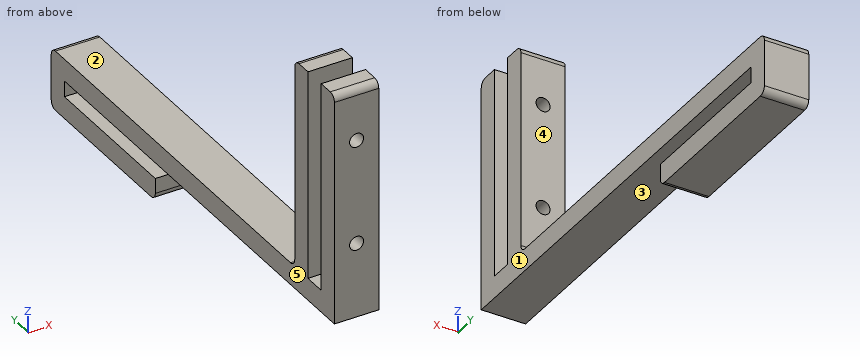
from build123d import *

# Parameters (mm, degrees)
SKETCH1_W           = 12.7
SKETCH1_H           = 66.548
BOSS_EXTRUDE1_DEPTH = 6.35
SKETCH2_W           = 12.7
SKETCH2_H           = 6.35
BOSS_EXTRUDE2_DEPTH = 6.35
SKETCH3_W           = 12.7
SKETCH3_H           = 66.548
BOSS_EXTRUDE3_DEPTH = 6.35
SKETCH4_W           = 12.7
SKETCH4_H           = 6.35
BOSS_EXTRUDE4_DEPTH = 117
SKETCH5_W           = 12.7
SKETCH5_H           = 6.35
BOSS_EXTRUDE5_DEPTH = 4.572
SKETCH6_W           = 12.7
SKETCH6_H           = 50
BOSS_EXTRUDE6_DEPTH = 6.35
BOSS_EXTRUDE7_DEPTH = 6.35
SKETCH9_R           = 2
CUT_EXTRUDE1_DEPTH  = 141.896738429
FILLET1_R           = 2
FILLET2_R           = 2


with BuildPart() as part:
    # Sketch1 → Boss-Extrude1 (new body)
    with BuildSketch(Plane(origin=(0, 0, 0), x_dir=(1, 0, 0), z_dir=(0, 1, 0))):
        with Locations((6.35, 33.274)):
            Rectangle(SKETCH1_W, SKETCH1_H)
    extrude(amount=BOSS_EXTRUDE1_DEPTH)

    # Sketch2 → Boss-Extrude2 (add)
    with BuildSketch(Plane(origin=(0, 6.35, 0), x_dir=(1, 0, 0), z_dir=(0, 1, 0))):
        with Locations((6.35, 63.373)):
            Rectangle(SKETCH2_W, SKETCH2_H)
    extrude(amount=BOSS_EXTRUDE2_DEPTH)

    # Sketch3 → Boss-Extrude3 (add)
    with BuildSketch(Plane(origin=(0, 12.7, 0), x_dir=(1, 0, 0), z_dir=(0, 1, 0))):
        with Locations((6.35, 33.274)):
            Rectangle(SKETCH3_W, SKETCH3_H)
    extrude(amount=BOSS_EXTRUDE3_DEPTH)

    # Sketch4 → Boss-Extrude4 (add)
    with BuildSketch(Plane(origin=(0, 19.05, 0), x_dir=(1, 0, 0), z_dir=(0, 1, 0))):
        with Locations((6.35, 63.373)):
            Rectangle(SKETCH4_W, SKETCH4_H)
    extrude(amount=BOSS_EXTRUDE4_DEPTH)

    # Sketch5 → Boss-Extrude5 (add)
    with BuildSketch(Plane(origin=(0, 0, -66.548), x_dir=(-1, 0, 0), z_dir=(0, 0, -1))):
        with Locations((-6.35, 132.875)):
            Rectangle(SKETCH5_W, SKETCH5_H)
    extrude(amount=BOSS_EXTRUDE5_DEPTH)

    # Sketch6 → Boss-Extrude6 (add)
    with BuildSketch(Plane(origin=(0, 0, -71.12), x_dir=(-1, 0, 0), z_dir=(0, 0, -1))):
        with Locations((-6.35, 111.05)):
            Rectangle(SKETCH6_W, SKETCH6_H)
    extrude(amount=BOSS_EXTRUDE6_DEPTH)

    # Sketch7 → Boss-Extrude7 (add)
    with BuildSketch(Plane(origin=(0, 6.35, 0), x_dir=(1, 0, 0), z_dir=(0, 1, 0))):
        with BuildLine():
            Line((12.7, 60.198), (0, 60.198))
            ThreePointArc((0, 60.198), (6.35, 60.107267194), (12.7, 60.198))
        make_face()
    extrude(amount=BOSS_EXTRUDE7_DEPTH)

    # Sketch9 → Cut-Extrude1 (cut, through all)
    with BuildSketch(Plane(origin=(0, 19.05, 0), x_dir=(1, 0, 0), z_dir=(0, 1, 0))):
        with Locations(Location((6.35, 45.099, 0), (0, 0, 270))):
            Circle(SKETCH9_R)
        with Locations(Location((6.35, 15.099, 0), (0, 0, 270))):
            Circle(SKETCH9_R)
    extrude(amount=-CUT_EXTRUDE1_DEPTH, mode=Mode.SUBTRACT)

    # Fillet1
    fillet1_edges = [part.edges().sort_by_distance(p)[0] for p in [
        (6.35, 19.05, 0),
        (6.35, 136.05, -60.198),
        (6.35, 0, 0),
        (6.35, 86.05, -77.47),
        (6.35, 136.05, -77.47),
    ]]
    fillet(fillet1_edges, radius=FILLET1_R)

    # Fillet2
    fillet2_edges = [part.edges().sort_by_distance(p)[0] for p in [
        (6.35, 19.05, -60.198),
    ]]
    fillet(fillet2_edges, radius=FILLET2_R)


solid = part.part
For this review, take the finished solid that the model builds, in its own axes (mm). Face numbers are marked on the shaded views. A direction names the side the tool comes from. Give positions to 0.01 mm unless a question says otherwise; leave off trailing zeros. Order: outer loops, then holes, each group sorted by start corner. A loop starts at its lowest first (then second) coordinate and runs counter-clockwise, first axis right, second up. Notation, with made-up numbers: (65, 0) -> (88, 0) arc R27 cw to (88, 35) -> close; hole circle Ø5 at (80.25, 67). An arc over 180 degrees is marked (long way). Write item = value, one per line.
1) We need section A-A, the plane y = 99. Give the boundary of the cut face in (x, z), and give its area (3 significant figures).
Findings:
outline = (0, -77.47) -> (12.7, -77.47) -> (12.7, -71.12) -> (0, -71.12) -> close; (0, -66.55) -> (12.7, -66.55) -> (12.7, -60.2) -> (0, -60.2) -> close
area = 161 mm^2
2) We need section D-D, the plane x = 6.35. Count the separate pieces of the cut face and the enclosed holes in it, and give its area (3 significant figures).
Findings:
separate_pieces = 5
enclosed_holes = 0
area = 1,870 mm^2
3) To check wall thickness, follow L1, parallel to Y at x = 9, z = -27; L2, parallel to Z at x = 7, y = 107. State the ranges of each line that lie inside material, in increasing order. Write a range as from..to.
Findings:
L1 = 0..6.35, 12.7..19.05
L2 = -77.47..-71.12, -66.55..-60.2
4) Draft analysis for pull direction Z (two halves, no side actions). For the marked faces 1, 2 and 3, state which applies: pulls with the +Z half, pulls with the -Z half, needs draft (parallel to the pull), parting line crosses it, or undercut.
Findings:
face_1 = needs draft
face_2 = pulls with the +Z half
face_3 = undercut
5) For the marked faces 4 and 5, list the 3-axis set-ups (+Z, -Z, +X, -X, +Y, -Y) from which the entire face can be reached by the end or side of a thin tool; tool diameter is ignored.
Findings:
face_4 = +Z, +X, -X, +Y
face_5 = +Z, -Z, -X, +Y, -Y
6) We need section B-B, the plane z = -48.5. Give the boundary of the cut face in (x, y).
Findings:
outline = (0, 0) -> (12.7, 0) -> (12.7, 6.35) -> (0, 6.35) -> close; (0, 12.7) -> (12.7, 12.7) -> (12.7, 19.05) -> (0, 19.05) -> close
7) We need section C-C, the plane y = 14. Give the boundary of the cut face in (x, z), and give its area (3 significant figures).
Findings:
outline = (0, -66.55) -> (12.7, -66.55) -> (12.7, 0) -> (0, 0) -> close; hole circle Ø4 at (6.35, -45.1); hole circle Ø4 at (6.35, -15.1)
area = 820 mm^2
8) Insertion check: pin 1 (4 mm diameter, centred on x = 9, z = -30.5, fed in from +Y); pin 2 (3.5 mm diameter, centred on x = 9, z = -73.5, fed in from -Y); pin 3 (6.5 mm diameter, centred on x = 4.5, y = 43.5, fed in from -Z); pin 4 (2.5 mm diameter, centred on x = 6.35, z = -45.099, fed in from +Y). Each pin has a flat end and moves straight along its axis. Give the tip position at first contact, or say it passes through.
Findings:
pin_1 = 19.05
pin_2 = 86.05
pin_3 = -66.55
pin_4 = through
